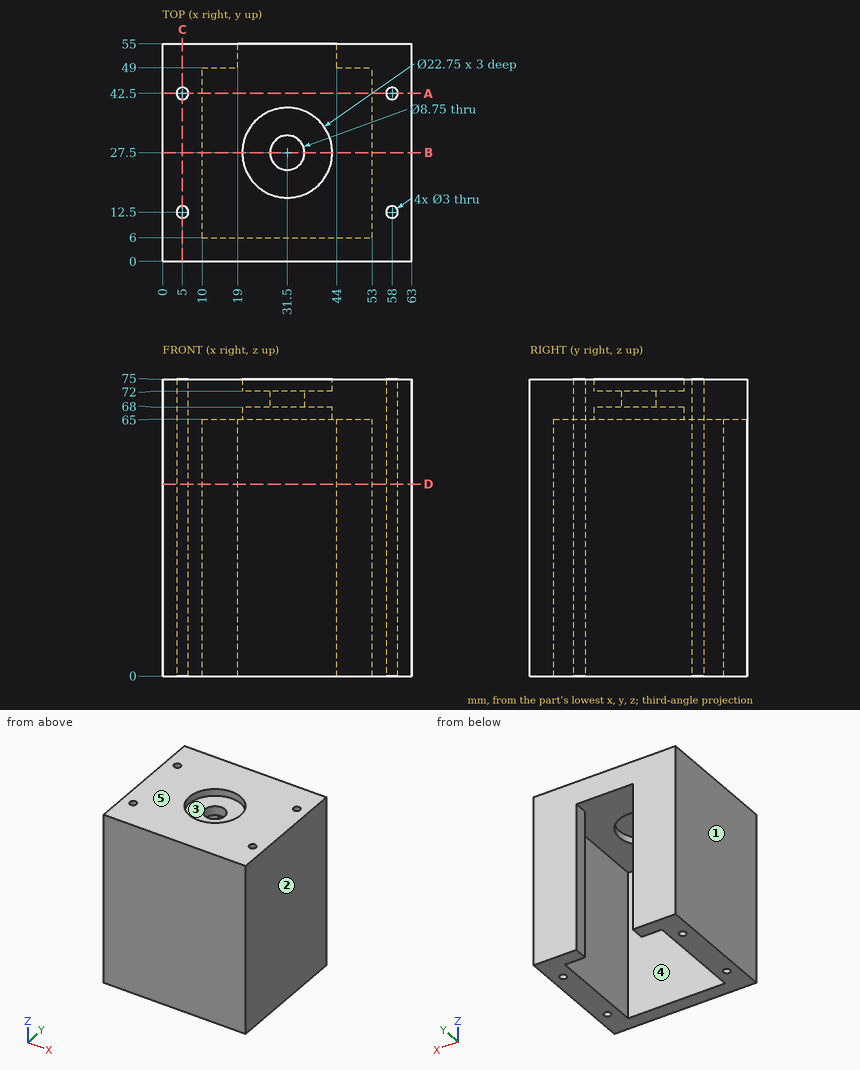
The figure shows three views and two pictorial views of one solid part (mm, origin at its lowest corner). Answer the questions. A direction names the side the tool comes from. Give positions to 0.01 mm unless a question says otherwise; leave off trailing zeros. Write each loop counter-clockwise with the first axis right and the second up, starting at its lowest first coordinate (ties: lowest second). Pieces come first, ordered by that corner, then holes. Notation, with made-up numbers: (-17, 83.5) - (-9, 83.5) arc R14 cw to (-9, 92.5) - close; hole circle Ø5 at (-6, 15). An arc over 180 degrees is marked (long way). Use CSV: the item, a comma, the result in double quotes. Start each with the question number.
Item 1: The part is cut by section B-B, the plane y = 27.5. Give the vertices of the cut face in (x, z) (3 decimals), and give its area (3 significant figures).
Item 2: The part is cut by section D-D, the plane z = 48.5. Give the vertices of the cut face in (x, y), and give its area (3 significant figures).
Item 3: Flat-ended cylindrical pins translate along their axes: P1, Ø2.5, axis at x = 5, y = 12.5, coming from the +Z side; P2, Ø10, axis at x = 50, z = 31.5, coming from the -Y side; P3, Ø10, axis at x = 31.5, y = 27.5, coming from the +Z side; P4, Ø21.5, axis at x = 28, y = 28, coming from the -Z side. Find the tip coordinate at first contact, or state that the pin passes through.
Item 4: For the marked faces 4 and 5, determine the directions among +Z, -Z, +X, -X, +Y, -Y from which every point of the face is accessible in a straight line to the end or side of a thin tool.
Item 5: The part is cut by section C-C, the plane x = 5. Give the vertices of the cut face in (y, z), and give its area (4 significant figures).
Item 6: Consider line 1 (Y direction, x = 58, z = 46); line 2 (X direction, y = 46.5, z = 25); line 3 (Y direction, x = 46, z = 22). Determine where each line is inside the solid, lowest interval first.
Item 7: The part is cut by section A-A, the plane y = 42.5. Give the vertices of the cut face in (x, z), and give its area (3 significant figures).
Item 8: The mould has two halves that part along X. Classify the marked faces 1, 2 and 3: pulls with the +X half, pulls with the -X half, needs draft (parallel to the pull), parting line crosses it, or undercut.
Taken from the geometry:
1,outline,"(0, 0) - (10, 0) - (10, 65) - (20.125, 65) - (20.125, 68) - (27.125, 68) - (27.125, 72) - (20.125, 72) - (20.125, 75) - (0, 75) - close; (35.875, 68) - (42.875, 68) - (42.875, 65) - (53, 65) - (53, 0) - (63, 0) - (63, 75) - (42.875, 75) - (42.875, 72) - (35.875, 72) - close"
1,area,"1,760 mm2"
2,outline,"(0, 0) - (63, 0) - (63, 55) - (44, 55) - (44, 49) - (53, 49) - (53, 6) - (10, 6) - (10, 49) - (19, 49) - (19, 55) - (0, 55) - close; hole circle Ø3 at (5, 12.5); hole circle Ø3 at (5, 42.5); hole circle Ø3 at (58, 12.5); hole circle Ø3 at (58, 42.5)"
2,area,"1,440 mm2"
3,P1,"through"
3,P2,"y = 0"
3,P3,"z = 72"
3,P4,"z = 65"
4,face 4,"-Z"
4,face 5,"+Z, +X, -X, +Y, -Y"
5,outline,"(0, 0) - (11, 0) - (11, 75) - (0, 75) - close; (14, 0) - (41, 0) - (41, 75) - (14, 75) - close; (44, 0) - (55, 0) - (55, 75) - (44, 75) - close"
5,area,"3,675 mm2"
6,line 1,"0 to 11, 14 to 41, 44 to 55"
6,line 2,"0 to 10, 53 to 63"
6,line 3,"0 to 6, 49 to 55"
7,outline,"(0, 0) - (3.5, 0) - (3.5, 75) - (0, 75) - close; (6.5, 0) - (10, 0) - (10, 65) - (53, 65) - (53, 0) - (56.5, 0) - (56.5, 75) - (6.5, 75) - close; (59.5, 0) - (63, 0) - (63, 75) - (59.5, 75) - close"
7,area,"1,480 mm2"
8,face 1,"pulls with the -X half"
8,face 2,"pulls with the +X half"
8,face 3,"undercut"
